from build123d import *

# Parameters (mm, degrees)
SKETCH_1_W          = 40.5
SKETCH_1_H          = 21
EXTRUDE_1_DEPTH     = 30.4
SKETCH_2_W          = 19
SKETCH_2_H          = 2.5
EXTRUDE_2_DEPTH     = 7
SKETCH_3_W          = 40.5
SKETCH_3_H          = 21
EXTRUDE_3_DEPTH     = 7
SKETCH_4_R          = 3
CUT_EXTRUDE_1_DEPTH = 7
SKETCH_5_R          = 4
SKETCH_5_R_2        = 2
EXTRUDE_4_DEPTH     = 4
FILLET_1_R          = 1
FILLET_2_R          = 1
FILLET_3_R          = 1
FILLET_4_R          = 1
FILLET_5_R          = 1
FILLET_6_R          = 1
FILLET_7_R          = 1
FILLET_8_R          = 1


with BuildPart() as part:
    # 草图1 → 凸台-拉伸1 (new body)
    with BuildSketch(Plane(origin=(0, 0, 0), x_dir=(1, 0, 0), z_dir=(0, 1, 0))):
        Rectangle(SKETCH_1_W, SKETCH_1_H)
    extrude(amount=EXTRUDE_1_DEPTH)

    # 草图2 → 凸台-拉伸2 (add)
    with BuildSketch(Plane(origin=(20.25, 0, 0), x_dir=(0, 0, -1), z_dir=(1, 0, 0))):
        with Locations((0, 29.15)):
            Rectangle(SKETCH_2_W, SKETCH_2_H)
    extrude_2 = extrude(amount=EXTRUDE_2_DEPTH)

    # 草图3 → 凸台-拉伸3 (add)
    with BuildSketch(Plane(origin=(0, 30.4, 0), x_dir=(1, 0, 0), z_dir=(0, 1, 0))):
        Rectangle(SKETCH_3_W, SKETCH_3_H)
    extrude(amount=EXTRUDE_3_DEPTH)

    # 草图4 → 切除-拉伸1 (cut)
    with BuildSketch(Plane(origin=(0, 30.4, 0), x_dir=(1, 0, 0), z_dir=(0, 1, 0))):
        with Locations((24.75, 5)):
            Circle(SKETCH_4_R)
        with Locations((24.75, -5)):
            Circle(SKETCH_4_R)
    cut_extrude_1 = extrude(amount=-CUT_EXTRUDE_1_DEPTH, mode=Mode.SUBTRACT)

    # 草图5 → 凸台-拉伸4 (add)
    with BuildSketch(Plane(origin=(0, 37.4, 0), x_dir=(1, 0, 0), z_dir=(0, 1, 0))):
        with Locations(Location((9.95, 0, 0), (0, 0, 270))):
            Circle(SKETCH_5_R)
        with Locations(Location((9.95, 0, 0), (0, 0, 270))):
            Circle(SKETCH_5_R_2, mode=Mode.SUBTRACT)
    extrude(amount=EXTRUDE_4_DEPTH)

    # 镜向2: 凸台-拉伸2, 切除-拉伸1 across plane
    add(extrude_2.mirror(Plane(origin=(0, 0, 0), x_dir=(0, 0, 1), z_dir=(1, 0, 0))))
    add(cut_extrude_1.mirror(Plane(origin=(0, 0, 0), x_dir=(0, 0, 1), z_dir=(1, 0, 0))), mode=Mode.SUBTRACT)

    # 圆角1
    fillet_1_edges = [part.edges().sort_by_distance(p)[0] for p in [
        (20.25, 18.7, -10.5),
    ]]
    fillet(fillet_1_edges, radius=FILLET_1_R - 0.0001)  # a hair under: the kernel refuses the full size

    # 圆角2
    fillet_2_edges = [part.edges().sort_by_distance(p)[0] for p in [
        (20.25, 18.7, 10.5),
    ]]
    fillet(fillet_2_edges, radius=FILLET_2_R - 0.0001)  # a hair under: the kernel refuses the full size

    # 圆角3
    fillet_3_edges = [part.edges().sort_by_distance(p)[0] for p in [
        (-20.25, 18.7, 10.5),
    ]]
    fillet(fillet_3_edges, radius=FILLET_3_R - 0.0001)  # a hair under: the kernel refuses the full size

    # 圆角4
    fillet_4_edges = [part.edges().sort_by_distance(p)[0] for p in [
        (-20.25, 18.7, -10.5),
    ]]
    fillet(fillet_4_edges, radius=FILLET_4_R - 0.0001)  # a hair under: the kernel refuses the full size

    # 圆角5
    fillet_5_edges = [part.edges().sort_by_distance(p)[0] for p in [
        (-27.25, 29.15, -9.5),
    ]]
    fillet(fillet_5_edges, radius=FILLET_5_R)

    # 圆角6
    fillet_6_edges = [part.edges().sort_by_distance(p)[0] for p in [
        (-27.25, 29.15, 9.5),
    ]]
    fillet(fillet_6_edges, radius=FILLET_6_R)

    # 圆角7
    fillet_7_edges = [part.edges().sort_by_distance(p)[0] for p in [
        (27.25, 29.15, 9.5),
    ]]
    fillet(fillet_7_edges, radius=FILLET_7_R)

    # 圆角8
    fillet_8_edges = [part.edges().sort_by_distance(p)[0] for p in [
        (27.25, 29.15, -9.5),
    ]]
    fillet(fillet_8_edges, radius=FILLET_8_R)


solid = part.part
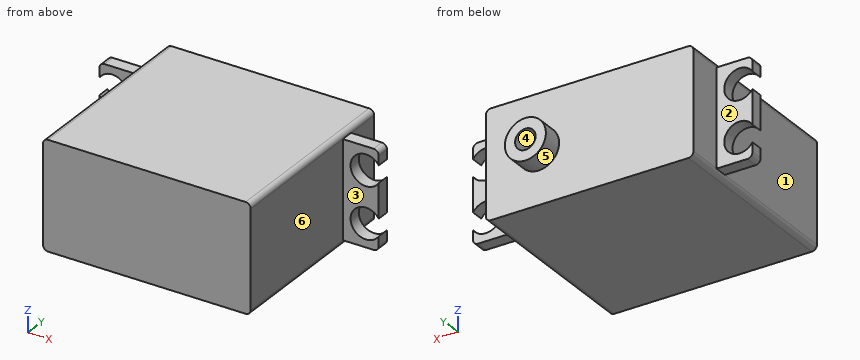
Build history of the part. All positions in model axes, mm. Face numbers are marked on the shaded views. A direction names the side the tool comes from. Round coordinates to 2 decimals unless told otherwise and drop trailing zeros. Order: outer loops, then holes, each group sorted by start corner. A loop starts at its lowest first (then second) coordinate and runs counter-clockwise, first axis right, second up. Notation, with made-up numbers: M -21.5,-24.75 L -11.5,-24.75 A18 cw -11.5,1.25 Z; hole C 18,52.5 d11. An arc over 180 degrees is marked long. Use CSV: the item, a comma, the result in double quotes. Start each with the question number.
(1) Cut at A-A on x = -24.75. List the corners of the cut face in (y, z), then the cut area to 3 significant figures.
(2) Cut at C-C on z = 5. List the corners of the cut face in (x, y), then the cut area to 3 significant figures.
(3) Cut at D-D on z = -2.75. List the corners of the cut face in (x, y).
(4) Drill centre lines: probe 1 along Z at (x, y) = (-24.75, 29.25); probe 2 along Z at (x, y) = (-24, 29); probe 3 along Y at (x, z) = (12, -4.25). Where is each one in solid material? Low to high.
(5) Mould opens along X. For the marked faces 4, 5 and 6 say: +X half, -X half, draft (parallel to the pull), parting line (faces both ways), or undercut.
(6) Tool access for the marked faces 1, 2 and 3: list every direction of +Z, -Z, +X, -X, +Y, -Y with a clear straight run to the whole face (end or side of a thin tool).
(7) Flat gauge pins, fed straight in: P1, Ø1, axis at y = 21.5, z = -1, coming from the +X side; P2, Ø6.5, axis at x = 2.5, z = -2.5, coming from the +Y side; P3, Ø9.5, axis at y = 13.5, z = 4, coming from the -X side. Where does each tip first touch, or does it go through?
Findings:
1,outline,"M 27.9,-9.5 L 30.4,-9.5 L 30.4,-8 L 27.9,-8 Z; M 27.9,-2 L 30.4,-2 L 30.4,2 L 27.9,2 Z; M 27.9,8 L 30.4,8 L 30.4,9.5 L 27.9,9.5 Z"
1,area,"17.5 mm^2"
2,outline,"M -21.75,27.9 L -20.25,27.9 L -20.25,0 L 20.25,0 L 20.25,27.9 L 21.75,27.9 L 21.75,30.4 L 20.25,30.4 L 20.25,37.4 L -20.25,37.4 L -20.25,30.4 L -21.75,30.4 Z"
2,area,"1,520 mm^2"
3,outline,"M -27.25,27.9 L -26.73,27.9 L -26.73,30.4 L -27.25,30.4 Z; M -22.77,27.9 L -20.25,27.9 L -20.25,0 L 20.25,0 L 20.25,27.9 L 22.77,27.9 L 22.77,30.4 L 20.25,30.4 L 20.25,37.4 L 12.85,37.4 L 12.85,41.4 L 7.05,41.4 L 7.05,37.4 L -20.25,37.4 L -20.25,30.4 L -22.77,30.4 Z; M 26.73,27.9 L 27.25,27.9 L 27.25,30.4 L 26.73,30.4 Z"
4,probe 1,"z = -9.5 to -8, -2 to 2, 8 to 9.5"
4,probe 2,"z = -9.5 to -7.9, -2.1 to 2.1, 7.9 to 9.5"
4,probe 3,"y = 0 to 37.4"
5,face 4,"undercut"
5,face 5,"parting line"
5,face 6,"+X half"
6,face 1,"+Z, -Z, -X"
6,face 2,"+Z, -Z, -X, +Y"
6,face 3,"+Z, -Z, +X, -Y"
7,P1,"stops at x = 20.25"
7,P2,"stops at y = 37.4"
7,P3,"stops at x = -20.25"
